Source: CAD feature listing. Evaluate the final solid. Frame: model axes, mm. A direction names the side the tool comes from. Give positions to 0.01 mm unless a question says otherwise; leave off trailing zeros. Loops run counter-clockwise (first coordinate to the right, second up) from the corner with the lowest first, then second, coordinate; pieces in that order, holes last. Notation, with made-up numbers: (18.25, 6.5) -> (24.25, 6.5) arc R16 ccw to (24.25, 35.5) -> close; hole circle Ø6 at (33.5, -13). An arc over 180 degrees is marked (long way). Return JSON: item names as keys, results as strings. Group by question number.
```python
from build123d import *

# Parameters (mm, degrees)
F0_W     = 55
F0_H     = 5
F1_DEPTH = 20
F2_R     = 9.5
F3_DEPTH = 5
F4_R     = 2
F5_DEPTH = 10.001
F6_R     = 4.5
F7_DEPTH = 7
F8_R     = 2
F9_DEPTH = 25


with BuildPart() as f1:
    # F0 (on Top) → F1 (new body)
    with BuildSketch(Plane.XY):
        with Locations((15.134409, 2.5)):
            Rectangle(F0_W, F0_H)
    extrude(amount=F1_DEPTH)

    # F2 (on face) → F3 (join)
    with BuildSketch(Plane.XZ):
        with Locations((15.134409, 10)):
            Circle(F2_R)
    extrude(amount=F3_DEPTH)

    # F4 (on face) → F5 (cut, through all)
    with BuildSketch(Plane.XZ.offset(5)):
        with Locations((15.134409, 10)):
            Circle(F4_R)
    extrude(amount=-F5_DEPTH, mode=Mode.SUBTRACT)

    # F6 (on face) → F7 (cut)
    with BuildSketch(Plane(origin=(0, 5, 0), x_dir=(-1, 0, 0), z_dir=(0, 1, 0))):
        with Locations((-15.134409, 10)):
            Circle(F6_R)
    extrude(amount=-F7_DEPTH, mode=Mode.SUBTRACT)

    # F8 (on face) → F9 (cut)
    with BuildSketch(Plane.XZ):
        with Locations((-4.365591, 10)):
            Circle(F8_R)
        with Locations((34.634409, 10)):
            Circle(F8_R)
    extrude(amount=-F9_DEPTH, mode=Mode.SUBTRACT)


solid = f1.part
```
1) Cut plane B-B on z = 10. Return loops of the section in (x, y), then the cut area to 3 significant figures.
2) Material intervals for line 1 (Y direction, x = -8.5, z = 16.5); line 2 (Z direction, x = 16.5, y = -4.25); line 3 (Z direction, x = 11, y = 4.5), sorted ascending.
3) Cut plane D-D on x = 4. Return loops of the section in (y, z), then the cut area to 3 significant figures.
4) Contact query for flat-ended pins moving along their axis: P1, Ø4, axis at y = -3.5, z = 18, coming from the -X side; P2, Ø4.5, axis at x = 15.13, z = 10, coming from the -Y side; P3, Ø1.5, axis at x = 21, y = -2.5, coming from the -Z side; P4, Ø5, axis at y = -3.5, z = 11.5, coming from the +X side. Output: stop coordinate, or through.
5) Mould query, pull axis Z, two halves, no side actions, for faces 4 (the face through (15, 3, 20)), 5 (the face through (15, 3, 0)), 6 (the face through (14, -2, 8)). Classes: released by +Z, released by -Z, zero draft, split by the parting line, or undercut.
6) Reachability of faces 1 (the face through (15, 5, 5)), 2 (the face through (19.63, 1.55, 10.2)), 3 (the face through (8.13, -2.46, 16.42)) from +Z, -Z, +X, -X, +Y, -Y: full face, straight path, thin tool, end or side. Return the list, or none.
7) Cut plane A-A on y = 2.25. Return loops of the section in (x, z), then the cut area to 3 significant figures.
8) Cut plane C-C on x = 34. Return loops of the section in (y, z).
Calculated:
{
 "1": {"outline": "(-12.37, 0) -> (-6.37, 0) -> (-6.37, 5) -> (-12.37, 5) -> close; (-2.37, 0) -> (5.63, 0) -> (5.63, -5) -> (13.13, -5) -> (13.13, -2) -> (10.63, -2) -> (10.63, 5) -> (-2.37, 5) -> close; (17.13, -5) -> (24.63, -5) -> (24.63, 0) -> (32.63, 0) -> (32.63, 5) -> (19.63, 5) -> (19.63, -2) -> (17.13, -2) -> close; (36.63, 0) -> (42.63, 0) -> (42.63, 5) -> (36.63, 5) -> close", "area": "255 mm2"},
 "2": {"line 1": "0 to 5", "line 2": "0.6 to 8.54, 11.46 to 19.4", "line 3": "0 to 8.22, 11.78 to 20"},
 "3": {"outline": "(0, 0) -> (5, 0) -> (5, 20) -> (0, 20) -> close", "area": "100 mm2"},
 "4": {"P1": "x = 7.77", "P2": "y = -5", "P3": "z = 1.99", "P4": "x = 24.63"},
 "5": {"face 4": "released by +Z", "face 5": "released by -Z", "face 6": "undercut"},
 "6": {"face 1": "+Z, -Z, +X, -X, +Y", "face 2": "+Y", "face 3": "-Y"},
 "7": {"outline": "(-12.37, 0) -> (42.63, 0) -> (42.63, 20) -> (-12.37, 20) -> close; hole circle Ø4 at (-4.37, 10); hole circle Ø9 at (15.13, 10); hole circle Ø4 at (34.63, 10)", "area": "1,010 mm2"},
 "8": {"outline": "(0, 0) -> (5, 0) -> (5, 8.1) -> (0, 8.1) -> close; (0, 11.9) -> (5, 11.9) -> (5, 20) -> (0, 20) -> close"}
}
